Check sheet for the modelled part. Datum: model origin and axes. Units: mm. Coordinates: 2 decimals unless noted, no trailing zeros. Order: outer loops, then holes, each group sorted by start corner. A loop starts at its lowest first (then second) coordinate and runs counter-clockwise, first axis right, second up.
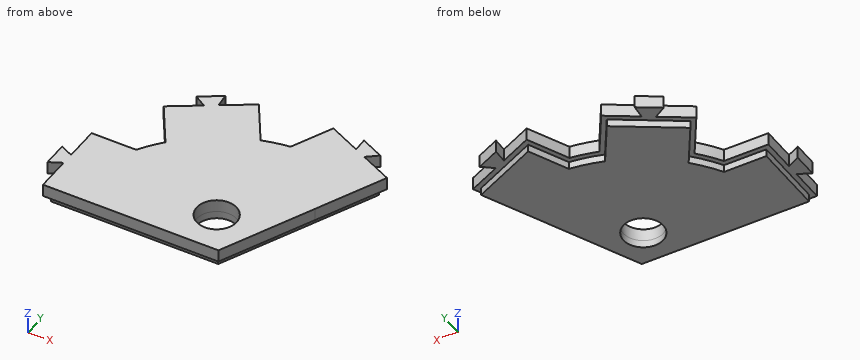
from build123d import *

# Parameters (mm, degrees)
F_1_1_2_2_6_BASE_SUJETADOR_OUTLINE_W   = 26
F_1_1_2_2_6_BASE_SUJETADOR_OUTLINE_H   = 28.884781413
F_1_1_2_2_6_BASE_SUJETADOR_OUTLINE_R   = 8
F_1_1_2_2_6_BASE_SUJETADOR_DEPTH       = 8
F_1_1_2_2_6_BASE_SUJETADOR_START       = 3
F_1_1_2_2_6_BASE_SUJETADOR_2_OUTLINE_W = 26
F_1_1_2_2_6_BASE_SUJETADOR_2_OUTLINE_H = 28.884781413
F_1_1_2_2_6_BASE_SUJETADOR_2_DEPTH     = 5
CROQUIS2_R                             = 8
SALIENTE_EXTRUIR1_DEPTH                = 5
CROQUIS3_R                             = 8
SALIENTE_EXTRUIR2_DEPTH                = 3


# Read off the part's stored shape, not the designer's step: 1.1.2.2.6_Base_Sujetador
with BuildPart() as part:
    # 1.1.2.2.6_Base_Sujetador outline → 1.1.2.2.6_Base_Sujetador (new body)
    with BuildSketch(Plane.XY):
        with Locations((-9.12411578, 30.387347077)):
            Rectangle(F_1_1_2_2_6_BASE_SUJETADOR_OUTLINE_W, F_1_1_2_2_6_BASE_SUJETADOR_OUTLINE_H)
        with Locations((-9.12411578, 30.387347076)):
            Circle(F_1_1_2_2_6_BASE_SUJETADOR_OUTLINE_R, mode=Mode.SUBTRACT)
    extrude(amount=F_1_1_2_2_6_BASE_SUJETADOR_DEPTH)

    # 1.1.2.2.6_Base_Sujetador 2 outline → 1.1.2.2.6_Base_Sujetador 2 (add)
    with BuildSketch(Plane.XY.offset(F_1_1_2_2_6_BASE_SUJETADOR_START)):
        Polygon((-24.12411578, 27.887347076), (-24.12411578, 13.94495637), (5.87588422, 13.94495637), (5.87588422, 46.829737783), (-24.12411578, 46.829737783), (-24.12411578, 32.887347076), (-29.12411578, 35.387347076), (-29.12411578, 25.387347076), align=None)
        with Locations((-9.12411578, 30.387347077)):
            Rectangle(F_1_1_2_2_6_BASE_SUJETADOR_2_OUTLINE_W, F_1_1_2_2_6_BASE_SUJETADOR_2_OUTLINE_H, mode=Mode.SUBTRACT)
    extrude(amount=F_1_1_2_2_6_BASE_SUJETADOR_2_DEPTH)

    # Croquis2 → Saliente-Extruir1 (add)
    # profile 1 of 2: a face of its own
    with BuildSketch(Plane.XY.offset(8)):
        Polygon((-6.240696441, 46.829737783), (-24.12411578, 46.829737783), (-24.12411578, 32.887347076), (-29.12411578, 35.387347076), (-29.12411578, 25.387347076), (-24.12411578, 27.887347076), (-24.12411578, 13.94495637), (5.87588422, 13.94495637), (5.87588422, 46.829737783), align=None)
    # profile 2 of 2: a face of its own
    with BuildSketch(Plane.XY.offset(8)):
        with BuildLine():
            ThreePointArc((0.348971375, 55.551526377), (-3.138373762, 51.336082183), (-6.240696441, 46.829737783))
            Line((-6.240696441, 46.829737783), (5.87588422, 46.829737783))
            Line((5.87588422, 46.829737783), (5.87588422, 13.94495637))
            Line((5.87588422, 13.94495637), (46.350842356, 13.94495637))
            Line((46.350842356, 13.94495637), (63.456298807, 50.627726109))
            Line((63.456298807, 50.627726109), (76.134846658, 77.81695972))
            Line((76.134846658, 77.81695972), (63.498749391, 83.709268645))
            Line((63.498749391, 83.709268645), (67.877610167, 87.184261926))
            Line((67.877610167, 87.184261926), (58.814532297, 91.410444543))
            Line((58.814532297, 91.410444543), (58.967210456, 85.822359953))
            Line((58.967210456, 85.822359953), (46.331113188, 91.714668878))
            Line((46.331113188, 91.714668878), (38.773253593, 75.506786672))
            ThreePointArc((38.773253593, 75.506786672), (33.378020355, 74.599590907), (28.083714716, 73.220506552))
            Line((28.083714716, 73.220506552), (17.505279389, 89.825323912))
            Line((17.505279389, 89.825323912), (5.746386333, 82.334082846))
            Line((5.746386333, 82.334082846), (5.168366906, 87.894289096))
            Line((5.168366906, 87.894289096), (-3.265547552, 82.521293012))
            Line((-3.265547552, 82.521293012), (1.529429104, 79.647584804))
            Line((1.529429104, 79.647584804), (-10.229463952, 72.156343738))
            Line((-10.229463952, 72.156343738), (0.348971375, 55.551526377))
        make_face()
        with Locations((35.87588422, 30.387347076)):
            Circle(CROQUIS2_R, mode=Mode.SUBTRACT)
    extrude(amount=-SALIENTE_EXTRUIR1_DEPTH)

    # Croquis3 → Saliente-Extruir2 (add)
    with BuildSketch(Plane(origin=(0, 0, 3), x_dir=(-1, 0, 0), z_dir=(0, 0, -1))):
        with BuildLine():
            Line((-73.476994561, 76.849580669), (-45.076701834, 15.94495637))
            Line((-45.076701834, 15.94495637), (22.12411578, 15.94495637))
            Line((22.12411578, 15.94495637), (22.12411578, 44.829737783))
            Line((22.12411578, 44.829737783), (5.12054128, 44.829737783))
            ThreePointArc((5.12054128, 44.829737783), (1.416566873, 50.296678088), (-2.865505455, 55.32367712))
            Line((-2.865505455, 55.32367712), (7.468081844, 71.544160063))
            Line((7.468081844, 71.544160063), (-16.893095714, 87.063941804))
            Line((-16.893095714, 87.063941804), (-27.226683013, 70.843458861))
            ThreePointArc((-27.226683013, 70.843458861), (-33.592373346, 72.599832764), (-40.112471141, 73.646344803))
            Line((-40.112471141, 73.646344803), (-47.298492239, 89.05681678))
            Line((-47.298492239, 89.05681678), (-73.476994561, 76.849580669))
        make_face()
        with Locations(Location((-35.87588422, 30.387347076, 0), (0, 0, 180))):
            Circle(CROQUIS3_R, mode=Mode.SUBTRACT)
    extrude(amount=SALIENTE_EXTRUIR2_DEPTH)


solid = part.part
(1) Go/stop test with flat-tipped pins: P1, Ø3, axis at x = 53, z = 5.5, coming from the -Y side; P2, Ø0.9, axis at y = 25.5, z = 1, coming from the -X side; P3, Ø0.9, axis at x = 9, z = 2, coming from the -Y side. Record where each tip stops, or that it passes through.
Filled in:
P1: stops at y = 24.99
P2: stops at x = -22.12
P3: stops at y = 15.94
(2) Cross-section at B-B (y = 23.5). Enter the section's corners in (x, z), and give its area (3 significant figures).
Filled in:
outline: (-24.12, 3) - (-22.12, 3) - (-22.12, 0) - (31.81, 0) - (31.81, 8) - (-24.12, 8) - close; (39.95, 0) - (48.6, 0) - (48.6, 3) - (50.81, 3) - (50.81, 8) - (39.95, 8) - close
area: 522 mm2
(3) Cross-section at A-A (x = -1). Enter the section's corners in (y, z), and give its area (3 significant figures).
Filled in:
outline: (13.94, 3) - (15.94, 3) - (15.94, 0) - (50.84, 0) - (50.84, 3) - (54.01, 3) - (54.01, 8) - (13.94, 8) - close; (57.67, 3) - (61.39, 3) - (61.39, 0) - (75.66, 0) - (75.66, 3) - (78.04, 3) - (78.04, 8) - (57.67, 8) - close; (81.16, 3) - (83.96, 3) - (83.96, 8) - (81.16, 8) - close
area: 464 mm2
(4) Cross-section at D-D (x = -20.5). Enter the section's corners in (y, z), and give its area (3 significant figures).
Filled in:
outline: (13.94, 3) - (15.94, 3) - (15.94, 0) - (44.83, 0) - (44.83, 3) - (46.83, 3) - (46.83, 8) - (13.94, 8) - close
area: 251 mm2
(5) Thickness scan on probe 1 along Y at (x, z) = (-0.5, 7.75); probe 2 along Y at (x, z) = (-0.5, 2); probe 3 along Y at (x, z) = (-18, 7.5). Record the ranges inside material, lowest first.
Filled in:
probe 1: y = 13.94 to 54.59, 56.88 to 78.35, 80.86 to 84.28
probe 2: y = 15.94 to 51.47, 60.61 to 75.98
probe 3: y = 13.94 to 46.83
(6) Cross-section at C-C (z = 6). Enter the section's corners in (x, y).
Filled in:
outline: (-29.12, 25.39) - (-24.12, 27.89) - (-24.12, 13.94) - (46.35, 13.94) - (76.13, 77.82) - (63.5, 83.71) - (67.88, 87.18) - (58.81, 91.41) - (58.97, 85.82) - (46.33, 91.71) - (38.77, 75.51) arc R62.03 ccw to (28.08, 73.22) - (17.51, 89.83) - (5.75, 82.33) - (5.17, 87.89) - (-3.27, 82.52) - (1.53, 79.65) - (-10.23, 72.16) - (0.35, 55.55) arc R62.03 ccw to (-6.24, 46.83) - (-24.12, 46.83) - (-24.12, 32.89) - (-29.12, 35.39) - close; hole circle Ø16 at (35.88, 30.39)
